from build123d import *

# Parameters (mm, degrees)
SKETCH1_W           = 50
SKETCH1_H           = 100
BOSS_EXTRUDE1_DEPTH = 5
CUT_EXTRUDE1_START  = -6
CUT_EXTRUDE1_DEPTH  = 7
FILLET1_R           = 5
SKETCH3_W           = 30.5
SKETCH3_H           = 30.5
CUT_EXTRUDE2_DEPTH  = 6
CUT_EXTRUDE3_START  = -6
SKETCH4_W           = 41.2
SKETCH4_H           = 3
CUT_EXTRUDE3_DEPTH  = 7


with BuildPart() as part:
    # Sketch1 → Boss-Extrude1 (new body)
    with BuildSketch(Plane(origin=(0, 0, 0), x_dir=(1, 0, 0), z_dir=(0, 1, 0))):
        Rectangle(SKETCH1_W, SKETCH1_H)
    extrude(amount=BOSS_EXTRUDE1_DEPTH)

    # Sketch2 → Cut-Extrude1 (cut)
    with BuildSketch(Plane(origin=(0, 5, 0), x_dir=(1, 0, 0), z_dir=(0, 1, 0)).offset(CUT_EXTRUDE1_START)):
        with BuildLine():
            Line((-17.5, -30.91), (17.5, -30.91))
            ThreePointArc((17.5, -30.91), (20.6, -34.01), (17.5, -37.11))
            Line((17.5, -37.11), (-17.5, -37.11))
            ThreePointArc((-17.5, -37.11), (-20.6, -34.01), (-17.5, -30.91))
        make_face()
    cut_extrude1 = extrude(amount=CUT_EXTRUDE1_DEPTH, mode=Mode.SUBTRACT)

    # Mirror1: Cut-Extrude1 across plane
    add(cut_extrude1.mirror(Plane.XY), mode=Mode.SUBTRACT)

    # Fillet1
    fillet1_edges = [part.edges().sort_by_distance(p)[0] for p in [
        (25, 2.5, 50),
        (-25, 2.5, 50),
        (-25, 2.5, -50),
        (25, 2.5, -50),
    ]]
    fillet(fillet1_edges, radius=FILLET1_R)

    # Sketch3 → Cut-Extrude2 (cut, through all)
    with BuildSketch(Plane(origin=(0, 5, 0), x_dir=(1, 0, 0), z_dir=(0, 1, 0))):
        Rectangle(SKETCH3_W, SKETCH3_H)
    extrude(amount=-CUT_EXTRUDE2_DEPTH, mode=Mode.SUBTRACT)

    # Sketch4 → Cut-Extrude3 (cut)
    with BuildSketch(Plane(origin=(0, 5, 0), x_dir=(1, 0, 0), z_dir=(0, 1, 0)).offset(CUT_EXTRUDE3_START)):
        with Locations((0, -19.775)):
            Rectangle(SKETCH4_W, SKETCH4_H)
        with Locations((0, -41.225)):
            Rectangle(SKETCH4_W, SKETCH4_H)
    cut_extrude3 = extrude(amount=CUT_EXTRUDE3_DEPTH, mode=Mode.SUBTRACT)

    # Mirror2: Cut-Extrude3 across plane
    add(cut_extrude3.mirror(Plane.XY), mode=Mode.SUBTRACT)


solid = part.part
Can you work these out from the model? Positions are in its coordinate system, mm. Coordinates: 2 decimals unless noted, no trailing zeros. Write each loop counter-clockwise with the first axis right and the second up, starting at its lowest first coordinate (ties: lowest second). Pieces come first, ordered by that corner, then holes. Notation, with made-up numbers: (61.25, 85.5) -> (91.25, 85.5) arc R8 cw to (91.25, 93.5) -> close; hole circle Ø7 at (61, 4). An arc over 180 degrees is marked (long way). Write each question's results on one line, items separated by ' | '. Start each with the question number.
Item 1: Thinking about a two-plate mould opening in Z: for faces 1 (the cylindrical face through (23, 3, 49)), 2 (the cylindrical face through (-24, 3, -48)), 3 (the flat face through (0, 2, -37.11)), which applies, released by +Z, released by -Z, zero draft, split by the parting line, or undercut?
Item 2: Please list where these lines run through material, in increasing order: probe 1 along X at (y, z) = (1.35, 6); probe 2 along X at (y, z) = (1.6, -41).
Item 3: If we section it at B-B, the plane x = -8: Count the separate pieces of the cut face and the enclosed holes in it, and give its area (4 significant figures).
Item 4: If we section it at A-A, the plane z = -34.01: Write out the boundary of the cut face in (x, y), and give its area (3 significant figures).
Item 5: If we section it at C-C, the plane z = -5.5: Write out the boundary of the cut face in (x, y), and give its area (3 significant figures).
Answer block:
1) face 1: released by +Z | face 2: released by -Z | face 3: undercut
2) probe 1: -25 to -15.25, 15.25 to 25 | probe 2: -25 to -20.6, 20.6 to 25
3) separate pieces: 8 | enclosed holes: 0 | area: 225.5 mm²
4) outline: (-25, 0) -> (-20.6, 0) -> (-20.6, 5) -> (-25, 5) -> close; (20.6, 0) -> (25, 0) -> (25, 5) -> (20.6, 5) -> close | area: 44.0 mm²
5) outline: (-25, 0) -> (-15.25, 0) -> (-15.25, 5) -> (-25, 5) -> close; (15.25, 0) -> (25, 0) -> (25, 5) -> (15.25, 5) -> close | area: 97.5 mm²
